For this review, use the dimensioned drawing (mm, ordinates from the lowest corner) and the shaded views. A direction names the side the tool comes from. Give positions to 0.01 mm unless a question says otherwise; leave off trailing zeros. Write each loop counter-clockwise with the first axis right and the second up, starting at its lowest first coordinate (ties: lowest second). Pieces come first, ordered by that corner, then holes.
1) Draft analysis for pull direction Y (two halves, no side actions). For the marked faces 3, 4, 5 and 6, state which applies: pulls with the +Y half, pulls with the -Y half, needs draft (parallel to the pull), parting line crosses it, or undercut.
2) Machinability: for the marked faces 1 and 2, which of the approach directions +Z, -Z, +X, -X, +Y, -Y give a long, thin tool a straight path to every point of the face, cutting with its end or side? Answer none if there is none.
3) We need section C-C on x = 419.5. Give the boundary of the cut face in (y, z), and give its area (3 significant figures).
4) We need section A-A on z = 426. Give the boundary of the cut face in (x, y).
5) We need section B-B on y = 542. Give the boundary of the cut face in (x, z) (1 decimal).
6) Wall thickness on line 1 along Y through (x, z) = (244, 356.5) (1 decimal); line 2 along Y through (x, z) = (249, 55); line 3 along X through (y, z) = (513.5, 431) (1 decimal): over which ranges is each line inside the solid? List them lowest first.
7) For P1, Ø1, axis at x = 328.5, y = 686, coming from the -Z side; P2, Ø1.5, axis at x = 413, z = 377.5, coming from the -Y side (1 decimal); P3, Ø1, axis at y = 324.5, z = 299, coming from the +X side, all flat-tipped, find the tip position at first contact; note any pin that passes through.
8) We need section D-D on y = 377.5. Give the boundary of the cut face in (x, z) (1 decimal).
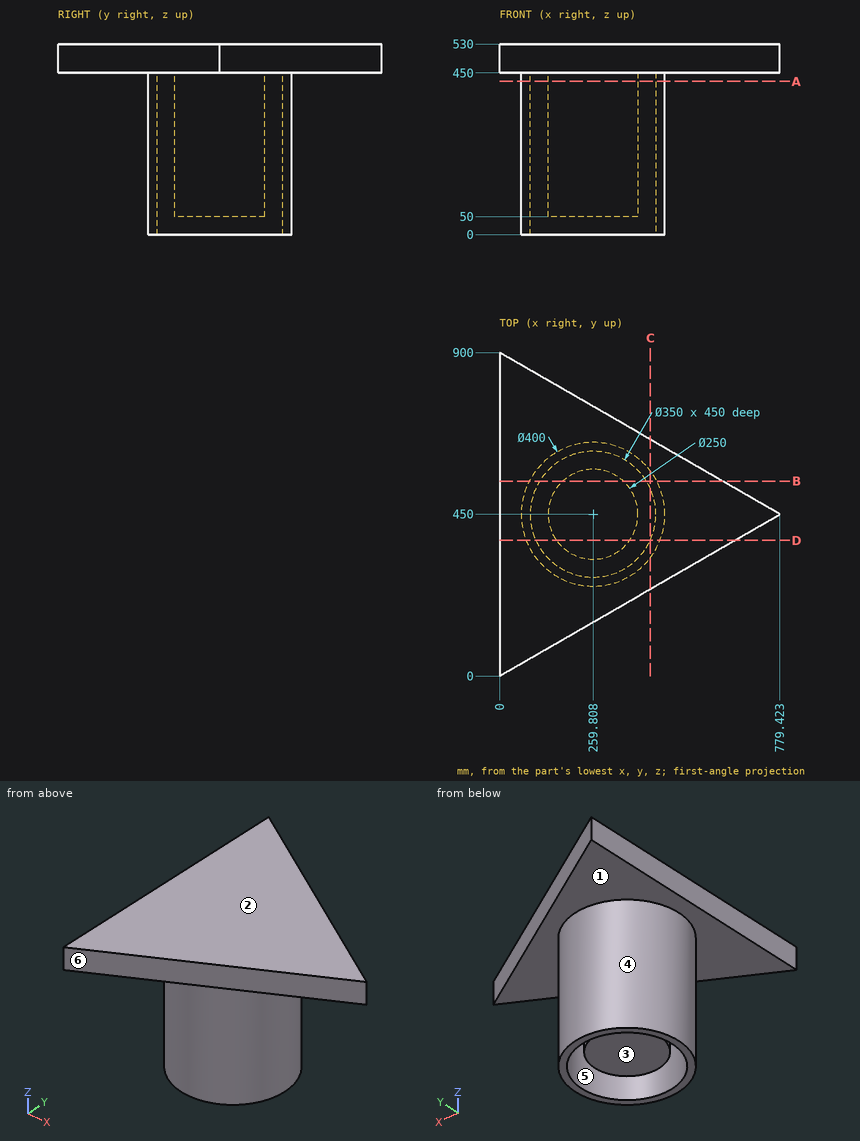
Results list:
1. face 3: undercut
1. face 4: parting line crosses it
1. face 5: undercut
1. face 6: pulls with the -Y half
2. face 1: -Z
2. face 2: +Z, +X, -X, +Y, -Y
3. outline: (242.2, 450) - (329.59, 450) - (329.59, 0) - (378.42, 0) - (378.42, 450) - (521.58, 450) - (521.58, 0) - (570.41, 0) - (570.41, 450) - (657.8, 450) - (657.8, 530) - (242.2, 530) - close
3. area: 77,200 mm2
4. outline: circle Ø400 at (259.81, 450); circle Ø250 at (259.81, 450); hole circle Ø350 at (259.81, 450)
5. outline: (0, 450) - (82.2, 450) - (82.2, 0) - (110.9, 0) - (110.9, 450) - (175.2, 450) - (175.2, 50) - (344.4, 50) - (344.4, 450) - (408.7, 450) - (408.7, 0) - (437.4, 0) - (437.4, 450) - (620.1, 450) - (620.1, 530) - (0, 530) - close
6. line 1: y = 250.6 to 275.7, 326 to 574, 624.3 to 649.4
6. line 2: y = 250.29 to 275.33, 325.47 to 574.53, 624.67 to 649.71
6. line 3: x = 70.2 to 96.7, 152.1 to 367.5, 422.9 to 449.5
7. P1: stops at z = 450
7. P2: stops at y = 320.5
7. P3: stops at x = 415.93
8. outline: (0, 450) - (73.4, 450) - (73.4, 0) - (100.5, 0) - (100.5, 450) - (158, 450) - (158, 50) - (361.6, 50) - (361.6, 450) - (419.1, 450) - (419.1, 0) - (446.2, 0) - (446.2, 450) - (653.8, 450) - (653.8, 530) - (0, 530) - close
